Part model, mm, in its own coordinate system. Face numbers are marked on the shaded views. A direction names the side the tool comes from. Give positions to 0.01 mm unless a question says otherwise; leave off trailing zeros. Write each loop counter-clockwise with the first axis right and the second up, starting at its lowest first coordinate (ties: lowest second). Pieces come first, ordered by that corner, then holes. Notation, with made-up numbers: (51, -20) - (92, -20) arc R22 ccw to (92, -10) - close; hole circle Ø1 at (-6.75, 45). An arc over 180 degrees is marked (long way). Answer as a JSON object with one key per item and string values. Group by question number.
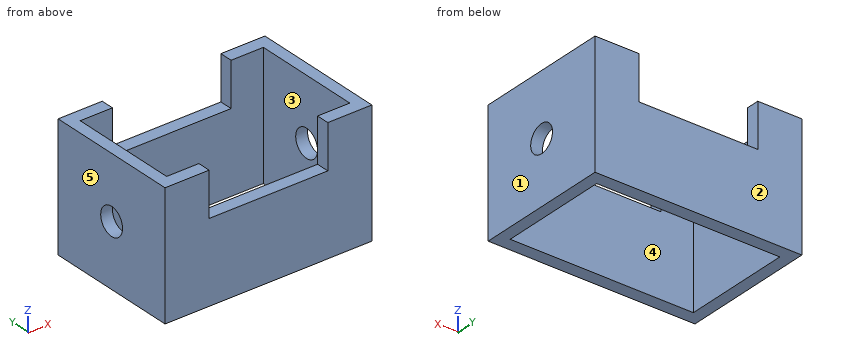
```python
from build123d import *

# Parameters (mm, degrees)
F0_W     = 104.681172
F0_H     = 95.793142
F0_R     = 10.65923
F1_DEPTH = 79.756
F2_W     = 141.289428
F2_H     = 84.574654
F3_DEPTH = 119.126
F5_DEPTH = 183.642


with BuildPart() as f1:
    # F0 (on Right) → F1 (new body, symmetric)
    with BuildSketch(Plane.YZ):
        Rectangle(F0_W, F0_H)
        Circle(F0_R, mode=Mode.SUBTRACT)
    extrude(amount=F1_DEPTH, both=True)

    # F2 (on face) → F3 (cut)
    with BuildSketch(Plane.XY.offset(47.896571)):
        Rectangle(F2_W, F2_H)
    extrude(amount=-F3_DEPTH, mode=Mode.SUBTRACT)

    # F4 (on face) → F5 (cut)
    with BuildSketch(Plane.XZ.offset(52.340586)):
        Polygon((45.769807, 47.896571), (0, 47.896571), (-45.769807, 47.896571), (-45.769807, 13.929941), (0, 13.929941), (45.769807, 13.929941), align=None)
    extrude(amount=-F5_DEPTH, mode=Mode.SUBTRACT)


solid = f1.part
```
1) Band-saw the part on A-A (z = 0). List the corners of the cut face in (x, y).
2) Band-saw the part on C-C (x = -64). List the corners of the cut face in (y, z).
3) Which spindle directions (+Z, -Z, +X, -X, +Y, -Y) get a long thin tool onto all of the face, cutting with end or side? Do the marked faces 4 and 5. Say none if no direction does.
4) Band-saw the part on B-B (z = -37.5). List the corners of the cut face in (x, y).
5) Probe line 1 (X direction, y = -13.5, z = -42.5); line 2 (Y direction, x = 76, z = 0); line 3 (Z direction, x = 75.25, y = 0). List the from-to ranges inside material, lowest first.
6) Drop flat-ended pins along their axis: P1, Ø19, axis at y = 0, z = 0, coming from the -X side; P2, Ø8, axis at x = 17.5, y = -45.5, coming from the +Z side. Give the stop position or say it passes through.
7) Band-saw the part on D-D (y = 0). List the corners of the cut face in (x, z), plus the area to 3 significant figures.
8) Mould opens along Y. For the marked faces 1, 2 and 3 say: pulls with the +Y half, pulls with the -Y half, needs draft (parallel to the pull), parting line crosses it, or undercut.
Verdict:
{
 "1": {"outline": "(-79.76, -52.34) - (79.76, -52.34) - (79.76, -10.66) - (70.64, -10.66) - (70.64, -42.29) - (-70.64, -42.29) - (-70.64, -10.66) - (-79.76, -10.66) - close; (-79.76, 10.66) - (-70.64, 10.66) - (-70.64, 42.29) - (70.64, 42.29) - (70.64, 10.66) - (79.76, 10.66) - (79.76, 52.34) - (-79.76, 52.34) - close"},
 "2": {"outline": "(-52.34, -47.9) - (-42.29, -47.9) - (-42.29, 47.9) - (-52.34, 47.9) - close; (42.29, -47.9) - (52.34, -47.9) - (52.34, 47.9) - (42.29, 47.9) - close"},
 "3": {"face 4": "+Z, -Z", "face 5": "+Z, -Z, -X, +Y, -Y"},
 "4": {"outline": "(-79.76, -52.34) - (79.76, -52.34) - (79.76, 52.34) - (-79.76, 52.34) - close; hole (-70.64, -42.29) - (70.64, -42.29) - (70.64, 42.29) - (-70.64, 42.29) - close"},
 "5": {"line 1": "-79.76 to -70.64, 70.64 to 79.76", "line 2": "-52.34 to -10.66, 10.66 to 52.34", "line 3": "-47.9 to -10.66, 10.66 to 47.9"},
 "6": {"P1": "through", "P2": "z = 13.93"},
 "7": {"outline": "(-79.76, -47.9) - (-70.64, -47.9) - (-70.64, -10.66) - (-79.76, -10.66) - close; (-79.76, 10.66) - (-70.64, 10.66) - (-70.64, 47.9) - (-79.76, 47.9) - close; (70.64, -47.9) - (79.76, -47.9) - (79.76, -10.66) - (70.64, -10.66) - close; (70.64, 10.66) - (79.76, 10.66) - (79.76, 47.9) - (70.64, 47.9) - close", "area": "1,360 mm2"},
 "8": {"face 1": "needs draft", "face 2": "pulls with the +Y half", "face 3": "undercut"}
}
